Work out the finished part from the listing and answer in its coordinate system (mm). Face numbers are marked on the shaded views. A direction names the side the tool comes from. Round coordinates to 2 decimals unless told otherwise and drop trailing zeros. Order: outer loops, then holes, each group sorted by start corner. A loop starts at its lowest first (then second) coordinate and runs counter-clockwise, first axis right, second up. Notation, with made-up numbers: (-17, 54.25) - (-11, 54.25) arc R24 cw to (-11, 71.25) - close; hole circle Ø10 at (84, 38). An arc over 180 degrees is marked (long way). Use CSV: the item, a comma, the result in double quotes.
from build123d import *

# Parameters (mm, degrees)
CROQUIS1_R              = 2.5
SALIENTE_EXTRUIR1_DEPTH = 5


with BuildPart() as part:
    # Croquis1 → Saliente-Extruir1 (new body)
    with BuildSketch(Plane.XY):
        with BuildLine():
            Line((5, -5), (5.590169944, -5))
            ThreePointArc((5.590169944, -5), (0, -7.5), (-5.590169944, -5))
            Line((-5.590169944, -5), (-5, -5))
            Line((-5, -5), (-5, 5))
            Line((-5, 5), (-5, 10))
            Line((-5, 10), (5, 10))
            Line((5, 10), (5, 5))
            Line((5, 5), (5, -5))
        make_face()
        Circle(CROQUIS1_R, mode=Mode.SUBTRACT)
    extrude(amount=SALIENTE_EXTRUIR1_DEPTH)


solid = part.part
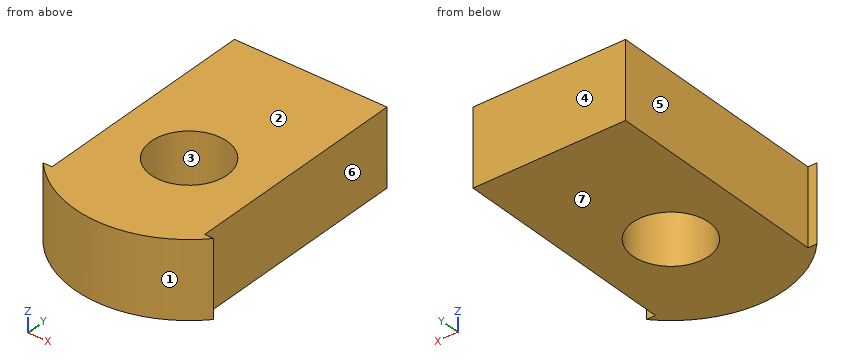
(1) Find the intervals of material crossed by L1, parallel to Y at x = 0, z = 1.6; L2, parallel to X at y = 7.25, z = 1.8; L3, parallel to Y at x = -2.75, z = 3.4, in increasing order. Write a range as from..to.
Findings below:
L1,"y = -7.5..-2.5, 2.5..10"
L2,"x = -5..5"
L3,"y = -6.98..10"
(2) The mould has two halves that part along Y. Classify the marked faces 1, 2, 3 and 4: released by +Y, released by -Y, zero draft, split by the parting line, or undercut.
Findings below:
face 1,"released by -Y"
face 2,"zero draft"
face 3,"undercut"
face 4,"released by +Y"
(3) Find section A-A (x = 0). Determine the outline of the cut face in (y, z), and give its area (3 significant figures).
Findings below:
outline,"(-7.5, 0) - (-2.5, 0) - (-2.5, 5) - (-7.5, 5) - close; (2.5, 0) - (10, 0) - (10, 5) - (2.5, 5) - close"
area,"62.5 mm²"
(4) For the marked faces 5, 6 and 7, determine the directions among +Z, -Z, +X, -X, +Y, -Y from which every point of the face is accessible in a straight line to the end or side of a thin tool.
Findings below:
face 5,"+Z, -Z, -X, +Y"
face 6,"+Z, -Z, +X, +Y"
face 7,"-Z, +X, -X, +Y, -Y"
(5) Find section D-D (y = -3). Determine the outline of the cut face in (x, z).
Findings below:
outline,"(-5, 0) - (5, 0) - (5, 5) - (-5, 5) - close"
(6) Find section C-C (y = 0). Determine the outline of the cut face in (x, z).
Findings below:
outline,"(-5, 0) - (-2.5, 0) - (-2.5, 5) - (-5, 5) - close; (2.5, 0) - (5, 0) - (5, 5) - (2.5, 5) - close"
(7) Each of these flat-tipped pins is pushed along its axis until it touches: pin 1 (2 mm diameter, centred on y = 8, z = 1.5, fed in from +X); pin 2 (1 mm diameter, centred on x = 2.5, y = 2, fed in from -Z); pin 3 (3 mm diameter, centred on x = 0, y = 0, fed in from -Z); pin 4 (2.5 mm diameter, centred on y = 6, z = 2, fed in from -X). Where does it stop, or does it pass through?
Findings below:
pin 1,"stops at x = 5"
pin 2,"stops at z = 0"
pin 3,"passes through"
pin 4,"stops at x = -5"
(8) Find section B-B (z = 0.5). Determine the outline of the cut face in (x, y), and give its area (3 significant figures).
Findings below:
outline,"(-5.59, -5) arc R7.5 ccw to (5.59, -5) - (5, -5) - (5, 10) - (-5, 10) - (-5, -5) - close; hole circle Ø5 at (0, 0)"
area,"150 mm²"
